Could you check a few things on this model? Use its own coordinates, in mm. A direction names the side the tool comes from. Give positions to 0.01 mm unless a question says otherwise; leave off trailing zeros. Write each loop counter-clockwise with the first axis right and the second up, starting at its lowest first coordinate (ties: lowest second). Pieces come first, ordered by that corner, then holes. Notation, with made-up numbers: (30, 59) - (57, 59) arc R23 ccw to (57, 73) - close; hole circle Ø8 at (-2.75, 54). An arc over 180 degrees is marked (long way). Use one line per item in the form item = value.
Autodesk Inventor part; units mm, degrees
ref_plane "Work Plane1" through (0, -9.6, 0) normal (-1, 0, 0) x (0, 0, 1)
ref_plane "YZ Plane" through (0, 0, 0) normal (1, 0, 0) x (0, 1, 0)
ref_plane "XZ Plane" through (0, 0, 0) normal (0, 1, 0) x (-1, 0, 0)
sketch "Base" plane through (0, 0, 0) normal (0, 0, 1) x (1, 0, 0)
  line L0 (-3.4, 9.6) -> (3.4, 9.6)
  line L1 (3.4, 9.6) -> (3.4, -9.6)
  line L2 (3.4, -9.6) -> (-3.4, -9.6)
  line L3 (-3.4, -9.6) -> (-3.4, 9.6)
  line L4 (-4.76, 0) -> (4.76, 0) construction
  line L5 (0, -13.44) -> (0, 13.44) construction
  point P0 (0, 0)
  point P1 (0, 9.6)
  point P2 (-3.4, 0)
  dimension "d0" = 6.8
  dimension "d1" = 19.2
extrude "BaseFeature" add sketch "Base" along normal blind 17.7
sketch "Mount" plane through (0, 0, 17.7) normal (0, 0, 1) x (1, 0, 0)
  line L0 (-4.8, 10.5) -> (4.8, 10.5)
  line L1 (4.8, 10.5) -> (4.8, -10.5)
  line L2 (4.8, -10.5) -> (-4.8, -10.5)
  line L3 (-4.8, -10.5) -> (-4.8, 10.5)
  line L4 (3.4, -9.6) -> (3.4, 9.6) construction
  line L5 (3.4, 0) -> (4.8, 0) construction
  line L6 (-3.4, -9.6) -> (3.4, -9.6) construction
  line L7 (0, -9.6) -> (0, -10.5) construction
  dimension "d13" = 9.6
  dimension "d14" = 21
extrude "MountFeature" add sketch "Mount" against normal blind 2
sketch "Sketch3" plane through (0, 0, 17.7) normal (0, 0, 1) x (1, 0, 0)
  line L0 (-2.3, -7.45) -> (2.3, -7.45)
  line L1 (-2.3, 7.45) -> (-2.3, -7.45)
  line L2 (2.3, 7.45) -> (-2.3, 7.45)
  line L3 (2.3, -7.45) -> (2.3, 7.45)
  line L4 (-4.8, 10.5) -> (-4.8, -10.5)
  line L5 (0, 0) -> (0, 10.5) construction
  line L6 (-4.8, 10.5) -> (4.8, 10.5)
  line L7 (-6.72, 0) -> (6.72, 0) construction
  point P0 (0, 7.45)
  point P1 (-2.3, 0)
  dimension "d22" = 14.9
  dimension "d23" = 4.6
extrude "Extrusion3" add sketch "Sketch3" along normal blind 4.2
fillet "Fillet4" radius 1 4 edges at (-2.3, 7.45, 19.8) (2.3, 7.45, 19.8) (-2.3, -7.45, 19.8) (2.3, -7.45, 19.8)
sketch "Sketch4" plane through (2.3, -7.45, 17.7) normal (1, 0, 0) x (0, 0, -1)
  line L0 (0, 0) -> (-4.2, 0)
  line L1 (-4.2, 14.9) -> (-4.2, 0)
  arc A0 (0, 0) -> (-4.2, 3.5647) centre (-50.9891, -55.8203) ccw
  line L2 (0, 0) -> (0, 14.9)
  arc A1 (-4.2, 3.5647) -> (0, 14.9) centre (-72.7661, 35.4157) ccw
  line L3 (0, 14.9) -> (-4.2, 14.9)
  point P0 (17.7, 7.45)
extrude "Extrusion4" cut sketch "Sketch4" against normal through all contours L0 L1 A0 | L1 L3 A1
fillet "Fillet1" radius 0.5 1 edges at (0, -3.8853, 21.9)
fillet "Fillet2" radius 1 4 edges at (4.8, -10.5, 16.7) (4.8, 10.5, 16.7) (-4.8, 10.5, 16.7) (-4.8, -10.5, 16.7)
fillet "Fillet3" radius 0.5 4 edges at (0, -10.5, 17.7) (4.8, 0, 17.7) (0, 10.5, 17.7) (-4.8, 0, 17.7)
sketch "Sketch6" plane through (-3.4, -9.6, 0) normal (-1, 0, 0) x (0, 0, 1)
  line L0 (0, 0) -> (0, 19.2) construction
  line L1 (0, 9.6) -> (0, 19.2)
  line L2 (0, 9.6) -> (15.7, 9.6) construction
  line L3 (15.7, 0) -> (15.7, 19.2)
  line L4 (0, 16.8553) -> (-7, 16.8553)
  line L5 (-7, 16.8553) -> (-7, 12.233)
  line L6 (-7, 12.233) -> (0, 12.233)
  line L7 (0, 12.233) -> (0, 16.8553)
  line L8 (0, 14.5441) -> (-7, 14.5441) construction
  line L9 (0, 2.3447) -> (-7, 2.3447)
  line L10 (-7, 2.3447) -> (-7, 6.967)
  line L11 (-7, 6.967) -> (0, 6.967)
  line L12 (0, 6.967) -> (0, 2.3447)
  dimension "d16" = 7
ref_plane "Work Plane1" through (0, -9.6, 0) normal (-1, 0, 0) x (0, 0, 1)
sketch "Sketch7" plane through (0, -9.6, 0) normal (-1, 0, 0) x (0, 0, 1)
  line L0 (0, 16.8553) -> (-7, 16.8553)
  line L1 (-7, 16.8553) -> (-7, 12.233)
  line L2 (-7, 12.233) -> (0, 12.233)
  line L3 (0, 19.2) -> (0, 0)
  line L4 (-7, 6.967) -> (0, 6.967)
  line L5 (-7, 2.3447) -> (-7, 6.967)
  line L6 (0, 2.3447) -> (-7, 2.3447)
  point P0 (0, 9.6)
extrude "Extrusion5" add sketch "Sketch7" along normal mid plane 1
chamfer "Chamfer1" distance 1 angle 45 4 edges at (0, 7.2553, -7) (0, 2.633, -7) (0, -2.633, -7) (0, -7.2553, -7)
properties part number "RockerSwitch"
1. For pin 1 (12.5 mm diameter, centred on y = 1.5, z = 10, fed in from -X); pin 2 (2 mm diameter, centred on x = -1, y = -2, fed in from -Z); pin 3 (2.5 mm diameter, centred on x = 0.5, y = -1.5, fed in from +Z); pin 4 (1.5 mm diameter, centred on y = 3.5, z = 0.5, fed in from +X), each with a flat end and sliding along its axis, tell me the tip position at first contact or that it passes through.
Response values:
pin_1 = -4.8
pin_2 = -6.23
pin_3 = 21.38
pin_4 = 3.4
2. Imagine slicing it at D-D, the plane y = 2. List the corners of the cut face in (x, z) for me, and give its area (3 significant figures).
Response values:
outline = (-4.8, 15.7) - (-3.4, 15.7) - (-3.4, 0) - (3.4, 0) - (3.4, 15.7) - (4.8, 15.7) - (4.8, 17.2) arc R0.5 ccw to (4.3, 17.7) - (2.3, 17.7) - (2.3, 19.46) - (-2.3, 19.46) - (-2.3, 17.7) - (-4.3, 17.7) arc R0.5 ccw to (-4.8, 17.2) - close
area = 134 mm²
3. If I drill on line 1 (X direction, y = 8.25, z = 0.5); line 2 (Z direction, x = -3.75, y = -5); line 3 (Z direction, x = -2.5, y = -1), over which ranges is the centre line in solid material (lowest first)? Write a range as from..to.
Response values:
line_1 = -3.4..3.4
line_2 = 15.7..17.7
line_3 = 0..17.7
4. Imagine slicing it at C-C, the plane x = 2.75. List the corners of the cut face in (y, z) for me, and give its area (3 significant figures).
Response values:
outline = (-10.5, 15.7) - (-9.6, 15.7) - (-9.6, 0) - (9.6, 0) - (9.6, 15.7) - (10.5, 15.7) - (10.5, 17.2) arc R0.5 ccw to (10, 17.7) - (-10, 17.7) arc R0.5 ccw to (-10.5, 17.2) - close
area = 343 mm²
5. Imagine slicing it at B-B, the plane y = -9. List the corners of the cut face in (x, z) for me, and give its area (3 significant figures).
Response values:
outline = (-4.8, 15.7) - (-3.4, 15.7) - (-3.4, 0) - (3.4, 0) - (3.4, 15.7) - (4.8, 15.7) - (4.8, 17.2) arc R0.5 ccw to (4.3, 17.7) - (-4.3, 17.7) arc R0.5 ccw to (-4.8, 17.2) - close
area = 126 mm²
6. Imagine slicing it at A-A, the plane z = -2.75. List the corners of the cut face in (x, y) for me, and give its area (3 significant figures).
Response values:
outline = (-0.5, -7.26) - (0.5, -7.26) - (0.5, -2.63) - (-0.5, -2.63) - close; (-0.5, 2.63) - (0.5, 2.63) - (0.5, 7.26) - (-0.5, 7.26) - close
area = 9.24 mm²
7. Which directions (+Z, -Z, +X, -X, +Y, -Y) give clear straight access to the entire face, cutting with the end or side of a thin tool? Please do faces 1 (the face through (0.007, 3.14, -6.507)), 2 (the face through (0, -9.6, 8)), 3 (the face through (0, 7.255, -3)), 4 (the face through (2.3, -2, 19)), 5 (the face through (0.5, 5, -4)).
Response values:
face_1 = -Z, +X, -X
face_2 = -Z, +X, -X, -Y
face_3 = -Z, +X, -X, +Y
face_4 = +Z, +X, +Y, -Y
face_5 = -Z, +X, +Y, -Y
